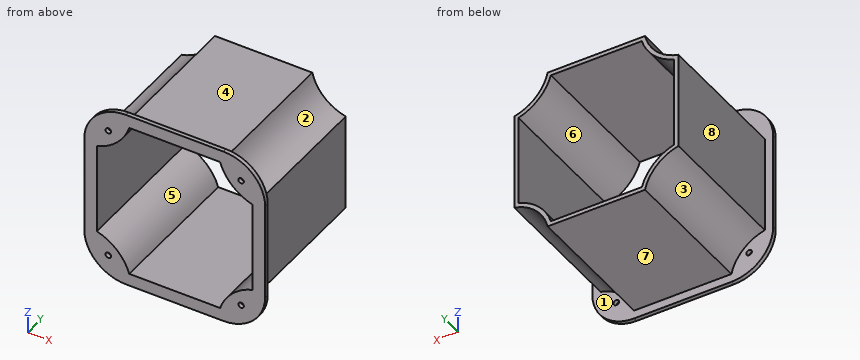
from build123d import *

# Parameters (mm, degrees)
SKETCH1_R                = 1
BOSS_EXTRUDE1_DEPTH      = 1.5
BOSS_EXTRUDE2_DEPTH      = 50
BOSS_EXTRUDE2_DEPTH_BACK = 1.5


with BuildPart() as part:
    # Sketch1 → Boss-Extrude1 (new body)
    with BuildSketch(Plane(origin=(0, 0, 0), x_dir=(1, 0, 0), z_dir=(0, 1, 0))):
        with BuildLine():
            Line((33.535245878, -16.168969585), (33.535245878, 18.831030415))
            ThreePointArc((33.535245878, 18.831030415), (29.141847596, 29.437632132), (18.535245878, 33.831030415))
            Line((18.535245878, 33.831030415), (-16.464754122, 33.831030415))
            ThreePointArc((-16.464754122, 33.831030415), (-27.07135584, 29.437632132), (-31.464754122, 18.831030415))
            Line((-31.464754122, 18.831030415), (-31.464754122, -16.168969585))
            ThreePointArc((-31.464754122, -16.168969585), (-27.07135584, -26.775571303), (-16.464754122, -31.168969585))
            Line((-16.464754122, -31.168969585), (18.535245878, -31.168969585))
            ThreePointArc((18.535245878, -31.168969585), (29.141847596, -26.775571303), (33.535245878, -16.168969585))
        make_face()
        with Locations((24.899206909, -22.532930616)):
            Circle(SKETCH1_R, mode=Mode.SUBTRACT)
        with Locations((-22.828715153, -22.532930616)):
            Circle(SKETCH1_R, mode=Mode.SUBTRACT)
        with Locations((-22.828715153, 25.194991445)):
            Circle(SKETCH1_R, mode=Mode.SUBTRACT)
        with Locations((24.899206909, 25.194991445)):
            Circle(SKETCH1_R, mode=Mode.SUBTRACT)
        with BuildLine():
            Line((18.535245878, -28.168969585), (-16.464754122, -28.168969585))
            ThreePointArc((-16.464754122, -28.168969585), (-20.723457919, -20.427673383), (-28.464754122, -16.168969585))
            Line((-28.464754122, -16.168969585), (-28.464754122, 18.831030415))
            ThreePointArc((-28.464754122, 18.831030415), (-20.723457919, 23.089734212), (-16.464754122, 30.831030415))
            Line((-16.464754122, 30.831030415), (18.535245878, 30.831030415))
            ThreePointArc((18.535245878, 30.831030415), (22.793949675, 23.089734212), (30.535245878, 18.831030415))
            Line((30.535245878, 18.831030415), (30.535245878, -16.168969585))
            ThreePointArc((30.535245878, -16.168969585), (22.793949675, -20.427673383), (18.535245878, -28.168969585))
        make_face(mode=Mode.SUBTRACT)
    extrude(amount=BOSS_EXTRUDE1_DEPTH)

    # Sketch2 → Boss-Extrude2 (add, two sides)
    with BuildSketch(Plane(origin=(0, 1.5, 0), x_dir=(1, 0, 0), z_dir=(0, 1, 0))) as boss_extrude2_sk:
        with BuildLine():
            Line((-28.464754122, 18.831030415), (-28.464754122, -16.168969585))
            ThreePointArc((-28.464754122, -16.168969585), (-20.723457919, -20.427673383), (-16.464754122, -28.168969585))
            Line((-16.464754122, -28.168969585), (18.535245878, -28.168969585))
            ThreePointArc((18.535245878, -28.168969585), (22.793949675, -20.427673383), (30.535245878, -16.168969585))
            Line((30.535245878, -16.168969585), (30.535245878, 18.831030415))
            ThreePointArc((30.535245878, 18.831030415), (22.793949675, 23.089734212), (18.535245878, 30.831030415))
            Line((18.535245878, 30.831030415), (-16.464754122, 30.831030415))
            ThreePointArc((-16.464754122, 30.831030415), (-20.723457919, 23.089734212), (-28.464754122, 18.831030415))
        make_face()
        with BuildLine():
            Line((29.035245878, -15.01127646), (29.035245878, 17.673337289))
            ThreePointArc((29.035245878, 17.673337289), (21.733289504, 22.02907404), (17.377552753, 29.331030415))
            Line((17.377552753, 29.331030415), (-15.307060997, 29.331030415))
            ThreePointArc((-15.307060997, 29.331030415), (-19.662797748, 22.02907404), (-26.964754122, 17.673337289))
            Line((-26.964754122, 17.673337289), (-26.964754122, -15.01127646))
            ThreePointArc((-26.964754122, -15.01127646), (-19.662797748, -19.367013211), (-15.307060997, -26.668969585))
            Line((-15.307060997, -26.668969585), (17.377552753, -26.668969585))
            ThreePointArc((17.377552753, -26.668969585), (21.733289504, -19.367013211), (29.035245878, -15.01127646))
        make_face(mode=Mode.SUBTRACT)
    extrude(amount=BOSS_EXTRUDE2_DEPTH)
    extrude(boss_extrude2_sk.sketch, amount=-BOSS_EXTRUDE2_DEPTH_BACK)


solid = part.part
Input: part model. Units: mm. Frame: model coordinates. Face numbers are marked on the shaded views. A direction names the side the tool comes from. Give positions to 0.01 mm unless a question says otherwise; leave off trailing zeros. Loops run counter-clockwise (first coordinate to the right, second up) from the corner with the lowest first, then second, coordinate; pieces in that order, holes last. Notation, with made-up numbers: (34.5, 79.25) -> (52.5, 79.25) arc R6 cw to (52.5, 84.25) -> close; hole circle Ø5 at (-26.5, 71.25). An arc over 180 degrees is marked (long way). Answer as a JSON object with one key per item and string values. Group by question number.
Item 1: Reachability of the marked faces 1, 2, 3, 4 and 5 from +Z, -Z, +X, -X, +Y, -Y: full face, straight path, thin tool, end or side. Return the list, or none.
Item 2: Cut plane B-B, the plane z = -22.5. Return the cut outline in (x, y).
Item 3: Pin query (flat end, axial travel): P1, Ø8, axis at x = 19.5, y = 22.5, coming from the +Z side; P2, Ø2.5, axis at x = 24.9, z = 22.53, coming from the +Y side; P3, Ø16.5, axis at x = -4, y = 30.5, coming from the -Z side. Return the tip coordinate at first contact, or that it passes through.
Item 4: Cut plane A-A, the plane y = 10.5. Return the cut outline in (x, z).
Item 5: Line query: probe 1 along X at (y, z) = (18, -14); probe 2 along Z at (x, y) = (-1.5, 18.5); probe 3 along Z at (x, y) = (19.5, 23.5). Output: solid intervals per line, ascending.
Item 6: Cut plane C-C, the plane x = 12. Return the cut outline in (y, z), and give its area (4 significant figures).
Item 7: Pull-direction query (Z, two-part tool) for the marked faces 6, 7 and 8; classes: released by +Z, released by -Z, zero draft, split by the parting line, or undercut.
Checks:
{
 "1": {"face 1": "+Y", "face 2": "+Z, +X, +Y", "face 3": "-Z, -X, +Y", "face 4": "+Z, +X, -X, +Y", "face 5": "+Y, -Y"},
 "2": {"outline": "(-31.01, 0) -> (-19.21, 0) -> (-19.21, 51.5) -> (-21.35, 51.5) -> (-21.35, 1.5) -> (-31.01, 1.5) -> close; (21.28, 0) -> (33.08, 0) -> (33.08, 1.5) -> (23.42, 1.5) -> (23.42, 51.5) -> (21.28, 51.5) -> close"},
 "3": {"P1": "stops at z = 28.17", "P2": "stops at y = 1.5", "P3": "stops at z = -30.83"},
 "4": {"outline": "(-28.46, -18.83) arc R15.85 cw to (-16.46, -30.83) -> (18.54, -30.83) arc R15.85 cw to (30.54, -18.83) -> (30.54, 16.17) arc R15.85 cw to (18.54, 28.17) -> (-16.46, 28.17) arc R15.85 cw to (-28.46, 16.17) -> close; hole (-26.96, -17.67) arc R17.35 cw to (-15.31, -29.33) -> (17.38, -29.33) arc R17.35 cw to (29.04, -17.67) -> (29.04, 15.01) arc R17.35 cw to (17.38, 26.67) -> (-15.31, 26.67) arc R17.35 cw to (-26.96, 15.01) -> close"},
 "5": {"probe 1": "x = -28.46 to -26.96, 29.04 to 30.54", "probe 2": "z = -30.83 to -29.33, 26.67 to 28.17", "probe 3": "z = -27.9 to -24.77, 22.11 to 25.24"},
 "6": {"outline": "(0, -33.83) -> (1.5, -33.83) -> (1.5, -30.83) -> (51.5, -30.83) -> (51.5, -29.33) -> (0, -29.33) -> close; (0, 26.67) -> (51.5, 26.67) -> (51.5, 28.17) -> (1.5, 28.17) -> (1.5, 31.17) -> (0, 31.17) -> close", "area": "163.5 mm²"},
 "7": {"face 6": "undercut", "face 7": "released by -Z", "face 8": "zero draft"}
}
